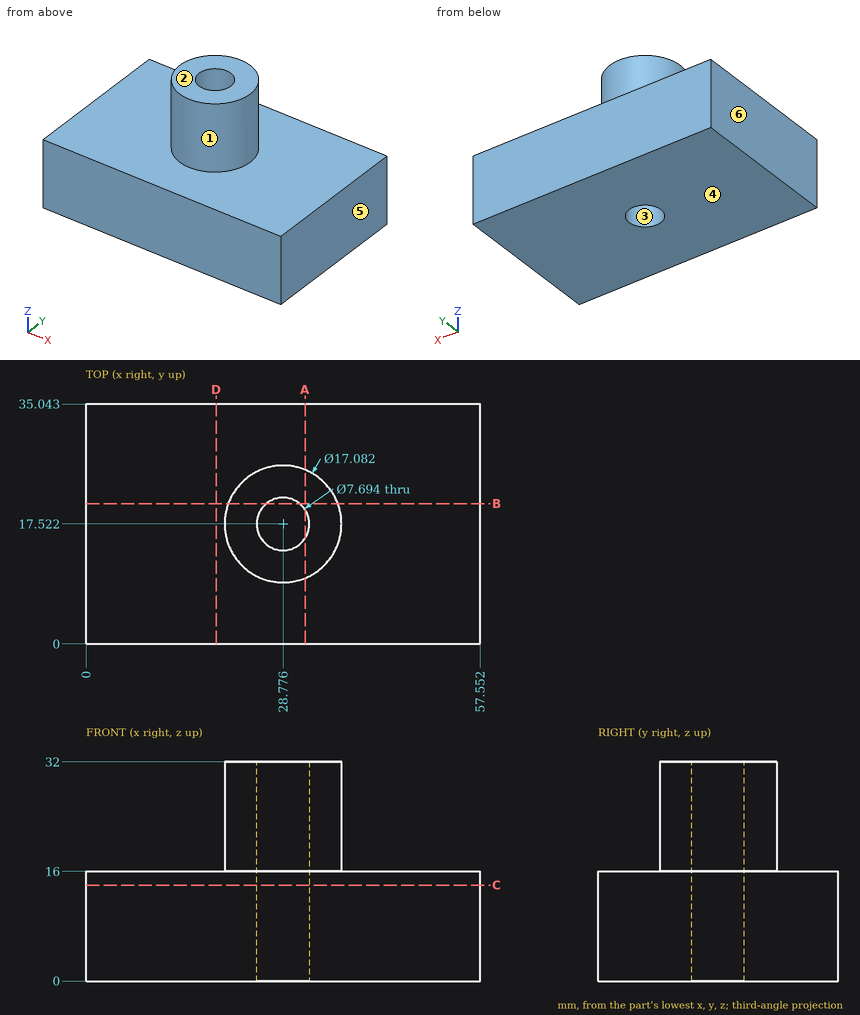
Source: three-view drawing plus pictorial views. Frame: mm from the lowest corner of the part. A direction names the side the tool comes from. Give positions to 0.01 mm unless a question says otherwise; leave off trailing zeros. Write each loop counter-clockwise with the first axis right and the second up, starting at its lowest first coordinate (ties: lowest second). Pieces come first, ordered by that corner, then holes. Notation, with made-up numbers: (10.5, 62.5) - (26.5, 62.5) arc R15 ccw to (26.5, 77.5) - close; hole circle Ø2 at (80.5, 19.25). An arc over 180 degrees is marked (long way). Write item = value, one per line. Start each with the question number.
Q1. Draft query along X for the marked faces 3, 4, 5 and 6. Return one class per face: +X half, -X half, draft (parallel to the pull), parting line (faces both ways), or undercut.
Q2. Cut plane D-D, the plane x = 19. Return loops of the section in (y, z), then the cut area to 3 significant figures.
Q3. Cut plane A-A, the plane x = 32. Return loops of the section in (y, z).
Q4. Material intervals for probe 1 along Z at (x, y) = (33.5, 9); probe 2 along Y at (x, z) = (32, 26.5) (1 decimal); probe 3 along Y at (x, z) = (26, 5.5) (1 decimal), sorted ascending.
Q5. Cut plane C-C, the plane z = 14. Return loops of the section in (x, y) (1 decimal), then the cut area to 3 significant figures.
Q6. Pin query (flat end, axial travel): pin 1 Ø4 at (y, z) = (16.5, 20) entering from +X; pin 2 Ø2 at (x, y) = (13.5, 6.5) entering from +Z. Return the tip coordinate at first contact, or that it passes through.
Q7. Reachability of the marked faces 1 and 2 from +Z, -Z, +X, -X, +Y, -Y: full face, straight path, thin tool, end or side. Return the list, or none.
Q8. Cut plane B-B, the plane y = 20.5. Return loops of the section in (x, z), then the cut area to 3 significant figures.
Computed values:
q1.face_3 = undercut
q1.face_4 = draft
q1.face_5 = +X half
q1.face_6 = -X half
q2.outline = (0, 0) - (35.04, 0) - (35.04, 16) - (0, 16) - close
q2.area = 561 mm²
q3.outline = (0, 0) - (15.42, 0) - (15.42, 32) - (9.61, 32) - (9.61, 16) - (0, 16) - close; (19.62, 0) - (35.04, 0) - (35.04, 16) - (25.43, 16) - (25.43, 32) - (19.62, 32) - close
q4.probe_1 = 0 to 16
q4.probe_2 = 9.6 to 15.4, 19.6 to 25.4
q4.probe_3 = 0 to 14.9, 20.2 to 35
q5.outline = (0, 0) - (57.6, 0) - (57.6, 35) - (0, 35) - close; hole circle Ø7.7 at (28.8, 17.5)
q5.area = 1,970 mm²
q6.pin_1 = 37.32
q6.pin_2 = 16
q7.face_1 = +Z
q7.face_2 = +Z, +X, -X, +Y, -Y
q8.outline = (0, 0) - (26.34, 0) - (26.34, 32) - (20.77, 32) - (20.77, 16) - (0, 16) - close; (31.21, 0) - (57.55, 0) - (57.55, 16) - (36.78, 16) - (36.78, 32) - (31.21, 32) - close
q8.area = 1,020 mm²
